Autodesk Inventor part; units mm, degrees
ref_plane "YZ Plane" through (0, 0, 0) normal (1, 0, 0) x (0, 1, 0)
ref_plane "XZ Plane" through (0, 0, 0) normal (0, 1, 0) x (-1, 0, 0)
ref_plane "XY Plane" through (0, 0, 0) normal (0, 0, 1) x (1, 0, 0)
sketch "Sketch1" plane through (0, 0, 0) normal (0, 0, 1) x (1, 0, 0)
  line L0 (0, 0) -> (18.5, 0)
  line L1 (18.5, 0) -> (18.5, 10)
  line L2 (18.5, 10) -> (0, 10)
  line L3 (0, 10) -> (0, 0)
  dimension "d0" = 18.5
  dimension "d1" = 10
extrude "Extrusion1" add sketch "Sketch1" along normal blind 3
sketch "Sketch2" plane through (0, 0, 0) normal (0, 0, -1) x (-1, 0, 0)
  line L0 (0, 0) -> (-18.5, 0)
  line L1 (0, 10) -> (0, 0)
  line L2 (-18.5, 10) -> (0, 10)
  line L3 (-18.5, 0) -> (-18.5, 10)
  line L4 (-5, 10) -> (-5, 0)
  dimension "d4" = 5
extrude "Extrusion2" cut sketch "Sketch2" against normal blind 1.7 contours L0 L3 L2 L4
sketch "Sketch3" plane through (0, 0, 3) normal (0, 0, 1) x (1, 0, 0)
  point P0 (0, 0)
  point P1 (2.5, 2)
  point P2 (2.5, 8)
  dimension "d7" = 6
  dimension "d8" = 2.5
  dimension "d9" = 2
hole "Hole1" at (2.5, 2, 3) at (2.5, 8, 3) direction (0, 0, -1) diameter 1.5 depth 8 tip angle 118 counterbore diameter 2.5 counterbore depth 1
sketch "Sketch4" plane through (0, 0, 1.7) normal (0, 0, -1) x (-1, 0, 0)
  circle A0 centre (-2.5, 2) radius 0.75
  point P0 (0, 0)
  point P1 (-11, 1)
  dimension "d18" = 8.5
  dimension "d26" = 1
hole "Hole2" at (11, 1, 1.7) direction (0, 0, 1) diameter 5 depth 0.5
properties part number "thumb_03 CMC bottom angle sensor holder"
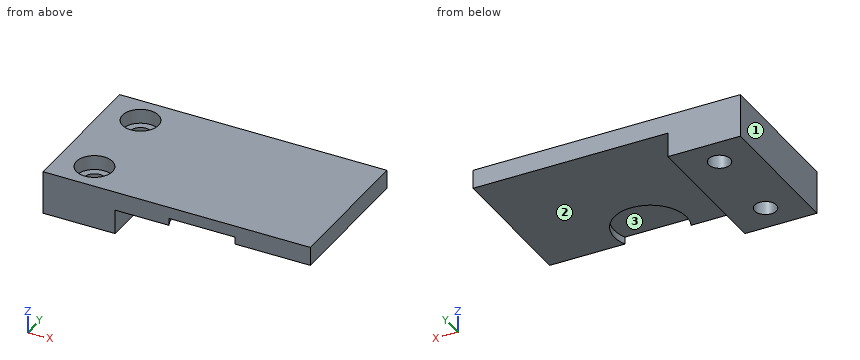
For this review, take the finished solid that the model builds, in its own axes (mm). Face numbers are marked on the shaded views. Round coordinates to 2 decimals unless told otherwise and drop trailing zeros. Write each loop counter-clockwise with the first axis right and the second up, starting at its lowest first coordinate (ties: lowest second). Pieces come first, ordered by that corner, then holes. Notation, with made-up numbers: (71, 16.25) - (107, 16.25) arc R27 cw to (107, 55.25) - close; hole circle Ø4 at (-8.5, -9.5). An arc over 180 degrees is marked (long way). Use CSV: the item, a comma, the result in double quotes.
1) Add section A-A on x = 2.5. Write out the cut boundary in (y, z), and give its area (3 significant figures).
Conclusion:
outline,"(0, 0) - (1.25, 0) - (1.25, 2) - (0.75, 2) - (0.75, 3) - (0, 3) - close; (2.75, 0) - (7.25, 0) - (7.25, 2) - (6.75, 2) - (6.75, 3) - (3.25, 3) - (3.25, 2) - (2.75, 2) - close; (8.75, 0) - (10, 0) - (10, 3) - (9.25, 3) - (9.25, 2) - (8.75, 2) - close"
area,"19.0 mm^2"
2) Add section B-B on y = 8. Write out the cut boundary in (x, z), and give its area (4 significant figures).
Conclusion:
outline,"(0, 0) - (1.75, 0) - (1.75, 2) - (1.25, 2) - (1.25, 3) - (0, 3) - close; (3.25, 0) - (5, 0) - (5, 1.7) - (18.5, 1.7) - (18.5, 3) - (3.75, 3) - (3.75, 2) - (3.25, 2) - close"
area,"27.05 mm^2"
3) The part is to be moulded in two halves that separate along X. For the marked faces 1, 2 and 3, say which applies: pulls with the +X half, pulls with the -X half, needs draft (parallel to the pull), parting line crosses it, or undercut.
Conclusion:
face 1,"pulls with the -X half"
face 2,"needs draft"
face 3,"undercut"
4) Wall thickness on line 1 along Y through (x, z) = (2.5, 1); line 2 along Y through (x, z) = (2.5, 2.65); line 3 along X through (y, z) = (2, 2.8): over which ranges is each line inside the solid? List them lowest first. Write a range as from..to.
Conclusion:
line 1,"y = 0..1.25, 2.75..7.25, 8.75..10"
line 2,"y = 0..0.75, 3.25..6.75, 9.25..10"
line 3,"x = 0..1.25, 3.75..18.5"
5) Clearance check with flat-ended pins moving along their axes: pin 1 Ø1.4 at (y, z) = (7, 0.5) entering from +X; pin 2 Ø2 at (x, y) = (2.5, 2) entering from +Z; pin 3 Ø3 at (x, y) = (11, 1) entering from -Z. State where each tip first meets the part, or that it passes through.
Conclusion:
pin 1,"stops at x = 5"
pin 2,"stops at z = 2"
pin 3,"stops at z = 2.2"
6) Add section D-D on x = 13. Write out the cut boundary in (y, z).
Conclusion:
outline,"(0, 2.2) - (2.5, 2.2) - (2.5, 1.7) - (10, 1.7) - (10, 3) - (0, 3) - close"
7) Add section C-C on z = 2.5. Write out the cut boundary in (x, y).
Conclusion:
outline,"(0, 0) - (18.5, 0) - (18.5, 10) - (0, 10) - close; hole circle Ø2.5 at (2.5, 2); hole circle Ø2.5 at (2.5, 8)"
